from build123d import *

# Parameters (mm, degrees)
F0_W      = 85
F0_H      = 56
F1_DEPTH  = 2
F2_R      = 1.25
F3_DEPTH  = 2
F4_R      = 2.5
F5_W      = 17
F5_H      = 15
F6_DEPTH  = 15
F7_W      = 13
F7_H      = 5
F8_DEPTH  = 15
F9_W      = 21
F9_H      = 16
F10_DEPTH = 13
F11_W     = 13
F11_H     = 8.5
F12_DEPTH = 15
F13_W     = 10
F13_H     = 1
F14_DEPTH = 3


with BuildPart() as f1:
    # F0 (on Top) → F1 (new body)
    with BuildSketch(Plane.XY):
        with Locations((40.44705, 38.563722)):
            Rectangle(F0_W, F0_H)
    extrude(amount=F1_DEPTH)

    # F2 (on face) → F3 (cut, through all)
    with BuildSketch(Plane.XY.offset(2)):
        with Locations((1.44705, 63.063722)):
            Circle(F2_R)
        with Locations((1.44705, 14.063722)):
            Circle(F2_R)
        with Locations((58.19705, 63.063722)):
            Circle(F2_R)
        with Locations((59.44705, 14.063722)):
            Circle(F2_R)
    extrude(amount=-F3_DEPTH, mode=Mode.SUBTRACT)

    # F4
    f4_edges = [f1.edges().sort_by_distance(p)[0] for p in [
        (82.94705, 10.563722, 1),
        (82.94705, 66.563722, 1),
        (-2.05295, 10.563722, 1),
        (-2.05295, 66.563722, 1),
    ]]
    fillet(f4_edges, radius=F4_R)

    # F5 (on face) → F6 (join)
    with BuildSketch(Plane.XY.offset(2)):
        with Locations((76.44705, 57.063722)):
            Rectangle(F5_W, F5_H)
        with Locations((76.44705, 39.063722)):
            Rectangle(F5_W, F5_H)
    extrude(amount=F6_DEPTH)

    # F7 (on face) → F8 (cut)
    with BuildSketch(Plane.YZ.offset(84.94705)):
        with Locations((39.063722, 13.5)):
            Rectangle(F7_W, F7_H)
        with Locations((39.063722, 5.5)):
            Rectangle(F7_W, F7_H)
        with Locations((57.063722, 13.5)):
            Rectangle(F7_W, F7_H)
        with Locations((57.063722, 5.5)):
            Rectangle(F7_W, F7_H)
    extrude(amount=-F8_DEPTH, mode=Mode.SUBTRACT)

    # F9 (on face) → F10 (join)
    with BuildSketch(Plane.XY.offset(2)):
        with Locations((74.44705, 21.063722)):
            Rectangle(F9_W, F9_H)
    extrude(amount=F10_DEPTH)

    # F11 (on face) → F12 (cut)
    with BuildSketch(Plane.YZ.offset(84.94705)):
        with Locations((21.063722, 8.75)):
            Rectangle(F11_W, F11_H)
    extrude(amount=-F12_DEPTH, mode=Mode.SUBTRACT)

    # F13 (on face) → F14 (join)
    with BuildSketch(Plane(origin=(-2.05295, 0, 0), x_dir=(0, -1, 0), z_dir=(-1, 0, 0))):
        with Locations((-38.563722, 0.5)):
            Rectangle(F13_W, F13_H)
    extrude(amount=F14_DEPTH)


solid = f1.part
Build history of the part. All positions in model axes, mm. A direction names the side the tool comes from. Give positions to 0.01 mm unless a question says otherwise; leave off trailing zeros. Loops run counter-clockwise (first coordinate to the right, second up) from the corner with the lowest first, then second, coordinate; pieces in that order, holes last. Notation, with made-up numbers: (22, 52) -> (41, 52) arc R3 cw to (41, 57) -> close; hole circle Ø7 at (30.5, 25.25). An arc over 180 degrees is marked (long way). Answer in a Markdown table with one row per item.
Item 1: Mould opens along X. For faces 6 (the flat face through (78, 45.564, 5)), 7 (the flat face through (67.947, 57, 9)), 8 (the cylindrical face through (60.024, 12.955, 1.014)) say: pulls with the +X half, pulls with the -X half, needs draft (parallel to the pull), parting line crosses it, or undercut.
Findings below:
| item | result |
|---|---|
| face 6 | needs draft |
| face 7 | pulls with the -X half |
| face 8 | undercut |
Item 2: Slice it at A-A on z = 6.75. Write the cut outline in (x, y).
Findings below:
| item | result |
|---|---|
| outline | (63.95, 13.06) -> (84.95, 13.06) -> (84.95, 14.56) -> (69.95, 14.56) -> (69.95, 27.56) -> (84.95, 27.56) -> (84.95, 29.06) -> (63.95, 29.06) -> close; (67.95, 31.56) -> (84.95, 31.56) -> (84.95, 32.56) -> (69.95, 32.56) -> (69.95, 45.56) -> (84.95, 45.56) -> (84.95, 46.56) -> (67.95, 46.56) -> close; (67.95, 49.56) -> (84.95, 49.56) -> (84.95, 50.56) -> (69.95, 50.56) -> (69.95, 63.56) -> (84.95, 63.56) -> (84.95, 64.56) -> (67.95, 64.56) -> close |
Item 3: Slice it at B-B on y = 55. Write the cut outline in (x, z).
Findings below:
| item | result |
|---|---|
| outline | (-2.05, 0) -> (82.95, 0) -> (82.95, 2) -> (84.95, 2) -> (84.95, 3) -> (69.95, 3) -> (69.95, 8) -> (84.95, 8) -> (84.95, 11) -> (69.95, 11) -> (69.95, 16) -> (84.95, 16) -> (84.95, 17) -> (67.95, 17) -> (67.95, 2) -> (-2.05, 2) -> close |
Item 4: Flat gauge pins, fed straight in: P1, Ø7.5, axis at y = 54, z = 11.5, coming from the -X side; P2, Ø2, axis at x = 84, y = 19, coming from the -Z side; P3, Ø2.5, axis at x = 81, z = 9.5, coming from the +Y side; P4, Ø1, axis at x = 62, z = 13.5, coming from the -Y side. Where does each tip first touch, or does it go through?
Findings below:
| item | result |
|---|---|
| P1 | stops at x = 67.95 |
| P2 | stops at z = 2 |
| P3 | stops at y = 64.56 |
| P4 | passes through |
Item 5: Probe line 1 along Y through (x, z) = (73.5, 9.25); line 2 along Z through (x, y) = (13.5, 15); line 3 along X through (y, z) = (44, 7.5). List the from-to ranges inside material, lowest first. Write a range as [from, to].
Findings below:
| item | result |
|---|---|
| line 1 | y = [13.06, 14.56], [27.56, 29.06], [31.56, 46.56], [49.56, 64.56] |
| line 2 | z = [0, 2] |
| line 3 | x = [67.95, 69.95] |
Item 6: Slice it at D-D on x = 44. Write the cut outline in (y, z).
Findings below:
| item | result |
|---|---|
| outline | (10.56, 0) -> (66.56, 0) -> (66.56, 2) -> (10.56, 2) -> close |
Item 7: Tool access for faces 1 (the flat face through (40, 10.564, 1)), 2 (the flat face through (78, 63.564, 13)), 3 (the flat face through (67.947, 39, 9)), 4 (the flat face through (74, 13.064, 8)), 5 (the cylindrical face through (-1.34, 11.315, 1.014)): list every direction of +Z, -Z, +X, -X, +Y, -Y with a clear straight run to the whole face (end or side of a thin tool).
Findings below:
| item | result |
|---|---|
| face 1 | +Z, -Z, +X, -X, -Y |
| face 2 | +X |
| face 3 | +Z, -X, +Y |
| face 4 | +Z, +X, -X, -Y |
| face 5 | +Z, -Z, -X, -Y |
Item 8: Slice it at C-C on x = 76.5. Give the number of separate pieces and of enclosed holes in the cut face, plus the area to 4 significant figures.
Findings below:
| item | result |
|---|---|
| separate pieces | 1 |
| enclosed holes | 5 |
| area | 399.5 mm² |
